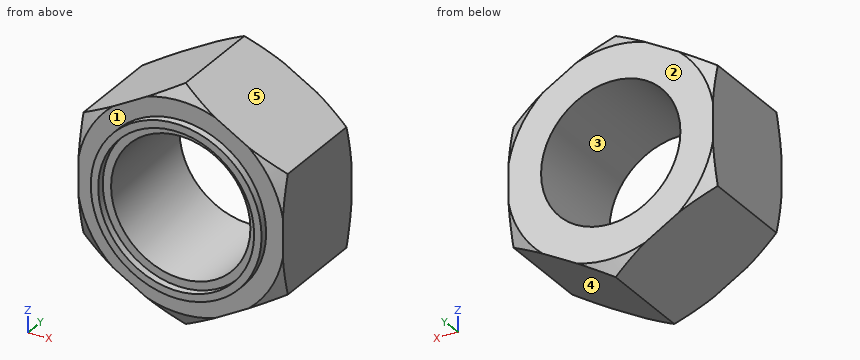
from build123d import *

# Parameters (mm, degrees)
BOSS_EXTRUDE1_DEPTH = 9.525
SKETCH4_W           = 11.9126
SKETCH4_H           = 19.05
SKETCH9_R           = 14.605
SKETCH9_R_2         = 13.335
BOSS_EXTRUDE2_DEPTH = 1.27


with BuildPart() as part:
    # Sketch1 → Boss-Extrude1 (new body, symmetric)
    with BuildSketch(Plane(origin=(0, 0, 0), x_dir=(1, 0, 0), z_dir=(0, 1, 0))):
        Polygon((17.4625, 10.081979076), (0, 20.163958151), (-17.4625, 10.081979076), (-17.4625, -10.081979076), (0, -20.163958151), (17.4625, -10.081979076), align=None)
    extrude(amount=BOSS_EXTRUDE1_DEPTH, both=True)

    # Sketch4 → Cut-Revolve1 (revolve, cut)
    with BuildSketch(Plane(origin=(0, 0, 0), x_dir=(0, 0, -1), z_dir=(1, 0, 0))):
        with Locations((-5.9563, 0)):
            Rectangle(SKETCH4_W, SKETCH4_H)
        Polygon((-17.78, -9.525), (-20.163958151, -8.14862112), (-20.163958151, -9.525), align=None)
        Polygon((-20.163958151, 9.525), (-17.78, 9.525), (-20.163958151, 8.14862112), align=None)
    revolve(axis=Axis((0, -9.525, 0), (0, 1, 0)), mode=Mode.SUBTRACT)

    # Sketch9 → Boss-Extrude2 (add)
    with BuildSketch(Plane.XZ.offset(9.525)):
        Circle(SKETCH9_R)
        Circle(SKETCH9_R_2, mode=Mode.SUBTRACT)
    extrude(amount=BOSS_EXTRUDE2_DEPTH)


solid = part.part
The listing builds one solid part. Answer for the finished solid, in the listing's coordinates (mm). Face numbers are marked on the shaded views. A direction names the side the tool comes from. Give positions to 0.01 mm unless a question says otherwise; leave off trailing zeros. Write each loop counter-clockwise with the first axis right and the second up, starting at its lowest first coordinate (ties: lowest second). Pieces come first, ordered by that corner, then holes.
Item 1: Flat-ended cylindrical pins translate along their axes: P1, Ø4, axis at x = 12.5, z = -15.5, coming from the -Y side; P2, Ø4, axis at x = 4, y = -1, coming from the -Z side; P3, Ø6, axis at y = -5.5, z = 15.5, coming from the +X side; P4, Ø6, axis at x = 1.5, y = -5.5, coming from the -Z side. Find the tip coordinate at first contact, or state that the pin passes through.
Item 2: Section B-B, the plane y = -6.75 is taken. Write down the section's boundary in (x, z), plus the area to 3 significant figures.
Item 3: Which of the six approach directions +Z, -Z, +X, -X, +Y, -Y give full straight-line access (tool end or side, diameter ignored) to the marked faces 1 and 2?
Item 4: Section A-A, the plane z = 0 is taken. Write down the section's boundary in (x, y) (1 decimal).
Item 5: Determine the mould class of the marked faces 3, 4 and 5 for opening direction Z: released by +Z, released by -Z, zero draft, split by the parting line, or undercut.
Item 6: Find the intervals of material crossed by line 1 along Z through (x, y) = (0, -10) (3 decimals); line 2 along X through (y, z) = (2, 0); line 3 along Y through (x, z) = (16, -1) (3 decimals), in increasing order.
Completed:
1. P1: passes through
1. P2: stops at z = -19.01
1. P3: stops at x = 13.27
1. P4: stops at z = -20.16
2. outline: (-17.46, -10.08) - (0, -20.16) - (17.46, -10.08) - (17.46, 10.08) - (0, 20.16) - (-17.46, 10.08) - close; hole circle Ø23.83 at (0, 0)
2. area: 611 mm2
3. face 1: -Y
3. face 2: +Z, -Z, +X, -X, +Y
4. outline: (-17.5, -9.5) - (-14.6, -9.5) - (-14.6, -10.8) - (-13.3, -10.8) - (-13.3, -9.5) - (-11.9, -9.5) - (-11.9, 9.5) - (-17.5, 9.5) - close; (11.9, -9.5) - (13.3, -9.5) - (13.3, -10.8) - (14.6, -10.8) - (14.6, -9.5) - (17.5, -9.5) - (17.5, 9.5) - (11.9, 9.5) - close
5. face 3: undercut
5. face 4: released by -Z
5. face 5: released by +Z
6. line 1: z = -14.605 to -13.335, 13.335 to 14.605
6. line 2: x = -17.46 to -11.91, 11.91 to 17.46
6. line 3: y = -9.525 to 9.525
